Geometry: see drawing. Coordinates: mm, zero at the bounding-box minimum. A direction names the side the tool comes from. Coordinates: 2 decimals unless noted, no trailing zeros. Write each loop counter-clockwise with the first axis right and the second up, starting at its lowest first coordinate (ties: lowest second). Pieces come first, ordered by that corner, then holes. Notation, with made-up numbers: M 75.5,-2 L 106.5,-2 A19 cw 106.5,16 Z; hole C 12.5,-13.75 d9. An arc over 180 degrees is marked long. Answer as CSV lines item,"result". Start each with the question number.
1. Section A-A on x = 69. Return the cut outline in (y, z), plus the area to 3 significant figures.
2. Reachability of the marked faces 1, 2, 3 and 4 from +Z, -Z, +X, -X, +Y, -Y: full face, straight path, thin tool, end or side. Return the list, or none.
3. Section C-C on y = 20.5. Return the cut outline in (x, z).
4. Line query: probe 1 along X at (y, z) = (4.5, 48.5); probe 2 along Z at (x, y) = (57, 24). Output: solid intervals per line, ascending. Write a range as [from, to].
5. Contact query for flat-ended pins moving along their axis: pin 1 Ø1 at (y, z) = (53, 27.5) entering from +X; pin 2 Ø12 at (y, z) = (15, 114) entering from -X; pin 3 Ø8 at (x, y) = (90, 62.5) entering from +Z. Output: stop coordinate, or through.
6. Section B-B on z = 76. Return the cut outline in (x, y), plus the area to 3 significant figures.
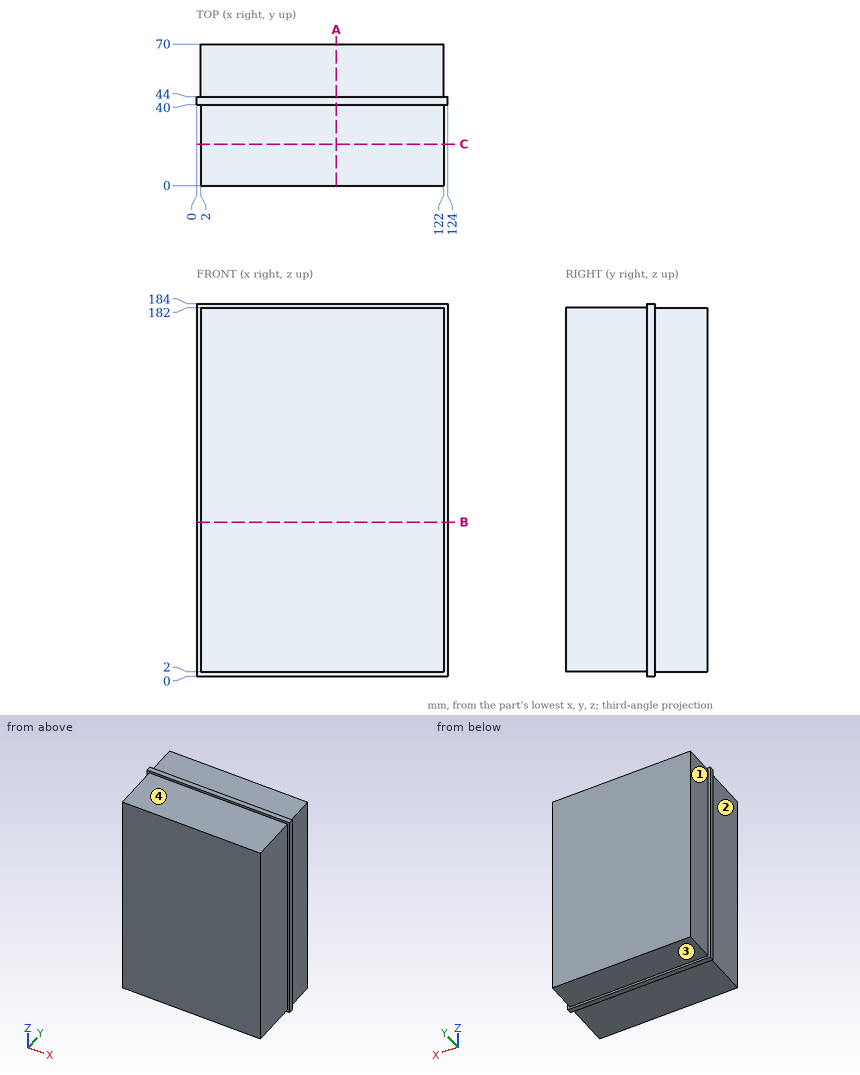
Values:
1,outline,"M 0,2 L 40,2 L 40,0 L 44,0 L 44,2 L 70,2 L 70,182 L 44,182 L 44,184 L 40,184 L 40,182 L 0,182 Z"
1,area,"12,600 mm²"
2,face 1,"+Z, -Z, -X, +Y"
2,face 2,"+Z, -Z, -X, -Y"
2,face 3,"-Z, +X, -X, +Y"
2,face 4,"+Z, +X, -X, -Y"
3,outline,"M 2,2 L 122,2 L 122,182 L 2,182 Z"
4,probe 1,"[2, 122]"
4,probe 2,"[2, 182]"
5,pin 1,"x = 122"
5,pin 2,"x = 2"
5,pin 3,"z = 182"
6,outline,"M 0,40 L 2,40 L 2,0 L 122,0 L 122,40 L 124,40 L 124,44 L 122,44 L 122,70 L 2,70 L 2,44 L 0,44 Z"
6,area,"8,420 mm²"
